Could you check a few things on this model? Use its own coordinates, in mm. Coordinates: 2 decimals unless noted, no trailing zeros. Loops run counter-clockwise (first coordinate to the right, second up) from the corner with the lowest first, then second, coordinate; pieces in that order, holes last.
from build123d import *

# Parameters (mm, degrees)
F0_R           = 37
F1_DEPTH       = 3
F3_D           = 3.3
F3_CSINK_D     = 6.72
F3_CSINK_ANGLE = 90


with BuildPart() as f1:
    # F0 (on Top) → F1 (new body)
    with BuildSketch(Plane.XY):
        Circle(F0_R)
    extrude(amount=F1_DEPTH)

    # F3 (through all)
    with Locations(Plane(origin=(0, 0, 0), x_dir=(1, 0, 0), z_dir=(0, 0, -1))):
        with Locations((-33.5, 0), (0, 33.5), (33.5, 0), (0, -33.5)):
            CounterSinkHole(F3_D / 2, F3_CSINK_D / 2, counter_sink_angle=F3_CSINK_ANGLE)


solid = f1.part
(1) We'd pull the mould along Y, two halves only. Please class faces 1 (the face through (-8.02, -36.12, 1.48)), 2 (the face through (-1, 1, 3)), 3 (the face through (0.215, 31.864, 2.364)): +Y half, -Y half, draft (parallel to the pull), parting line (faces both ways), or undercut.
Answers:
face 1: parting line
face 2: draft
face 3: undercut
(2) I need wall thicknesses on probe 1 along Y at (x, z) = (0, 2.4); probe 2 along Y at (x, z) = (33, 1.2); probe 3 along Y at (x, z) = (-33.5, 2.75). Which ranges of each line are inside material? Lowest first, please.
Answers:
probe 1: y = -37 to -35.15, -31.85 to 31.85, 35.15 to 37
probe 2: y = -16.73 to -2.1, 2.1 to 16.73
probe 3: y = -15.71 to -1.65, 1.65 to 15.71
(3) Imagine slicing it at A-A, the plane x = 0. Write out the boundary of the cut face in (y, z), and give its area (3 significant figures).
Answers:
outline: (-37, 0) - (-36.86, 0) - (-35.15, 1.71) - (-35.15, 3) - (-37, 3) - close; (-31.85, 1.71) - (-30.14, 0) - (30.14, 0) - (31.85, 1.71) - (31.85, 3) - (-31.85, 3) - close; (35.15, 1.71) - (36.86, 0) - (37, 0) - (37, 3) - (35.15, 3) - close
area: 196 mm2
(4) Imagine slicing it at C-C, the plane z = 1.1. Write out the boundary of the cut face in (x, y).
Answers:
outline: circle Ø74 at (0, 0); hole circle Ø4.52 at (-33.5, 0); hole circle Ø4.52 at (0, -33.5); hole circle Ø4.52 at (0, 33.5); hole circle Ø4.52 at (33.5, 0)
(5) Imagine slicing it at D-D, the plane x = 33.5. Write out the boundary of the cut face in (y, z).
Answers:
outline: (-15.71, 0) - (-3.36, 0) - (-1.65, 1.71) - (-1.65, 3) - (-15.71, 3) - close; (1.65, 1.71) - (3.36, 0) - (15.71, 0) - (15.71, 3) - (1.65, 3) - close
(6) For pin 1 (1.5 mm diameter, centred on y = -12, z = 0.5, fed in from +X); pin 2 (4 mm diameter, centred on x = 0, y = 33.5, fed in from -Z); pin 3 (4.5 mm diameter, centred on x = -33.5, y = 0, fed in from +Z); pin 4 (1 mm diameter, centred on y = -2, z = 1, fed in from +X), each with a flat end and sliding along its axis, tell me the tip position at first contact or that it passes through.
Answers:
pin 1: stops at x = 35.25
pin 2: stops at z = 1.36
pin 3: stops at z = 3
pin 4: stops at x = 36.97
